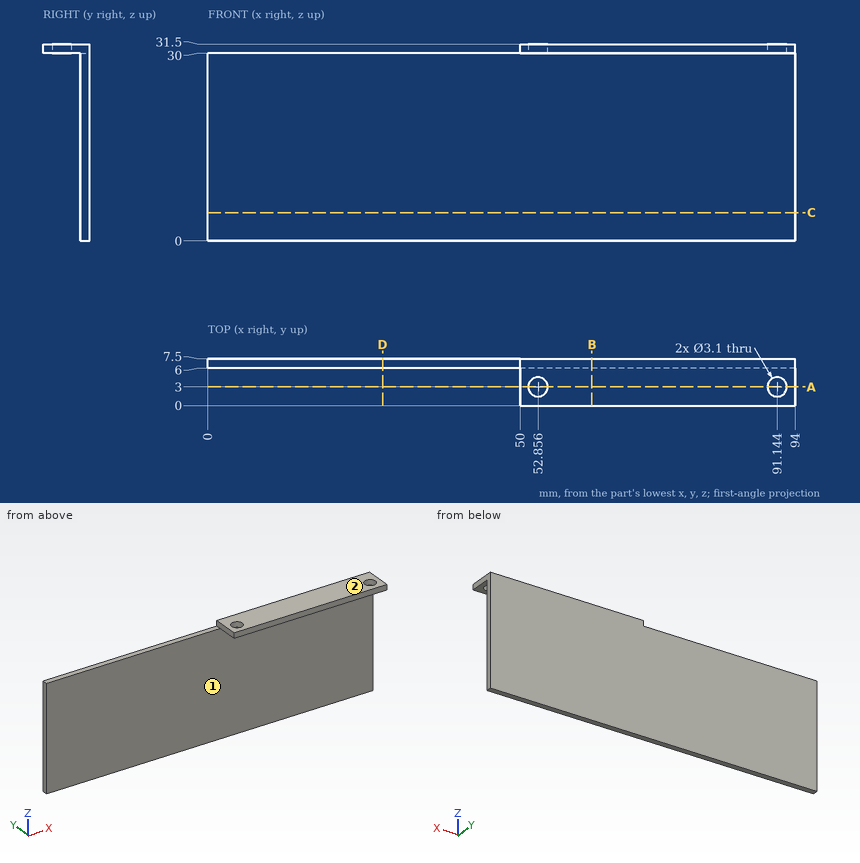
Geometry: see drawing. Coordinates: mm, zero at the bounding-box minimum. A direction names the side the tool comes from. Coordinates: 2 decimals unless noted, no trailing zeros. Loops run counter-clockwise (first coordinate to the right, second up) from the corner with the lowest first, then second, coordinate; pieces in that order, holes last.
(1) Section C-C on z = 4.5. Return the cut outline in (x, y), then the cut area to 3 significant figures.
(2) Set-up query: the marked faces 1 and 2. Return all of +Z, -Z, +X, -X, +Y, -Y with unobstructed straight access to the full face (end or side cutting, diameter ignored); none if empty.
(3) Section B-B on x = 61.5. Return the cut outline in (y, z).
(4) First-contact query: pin 1 Ø2 at (x, y) = (59, 4.5) entering from -Z; pin 2 Ø0.8 at (y, z) = (3, 30.5) entering from -X; pin 3 Ø10 at (x, z) = (26.5, 12.5) entering from -Y. Flat tips, straight axial feed; report the tip coordinate or a pass-through.
(5) Section A-A on y = 3. Return the cut outline in (x, z).
(6) Material intervals for probe 1 along Y at (x, z) = (6, 2.5); probe 2 along Z at (x, y) = (77, 1.5); probe 3 along Z at (x, y) = (22, 6.5), sorted ascending.
(7) Section D-D on x = 28. Return the cut outline in (y, z), then the cut area to 3 significant figures.
Data:
1. outline: (0, 6) - (94, 6) - (94, 7.5) - (0, 7.5) - close
1. area: 141 mm2
2. face 1: -Z, +X, -X, -Y
2. face 2: +Z, +X, -X, +Y, -Y
3. outline: (0, 30) - (6, 30) - (6, 0) - (7.5, 0) - (7.5, 31.5) - (0, 31.5) - close
4. pin 1: stops at z = 30
4. pin 2: stops at x = 50
4. pin 3: stops at y = 6
5. outline: (50, 30) - (51.31, 30) - (51.31, 31.5) - (50, 31.5) - close; (54.41, 30) - (89.59, 30) - (89.59, 31.5) - (54.41, 31.5) - close; (92.69, 30) - (94, 30) - (94, 31.5) - (92.69, 31.5) - close
6. probe 1: y = 6 to 7.5
6. probe 2: z = 30 to 31.5
6. probe 3: z = 0 to 30
7. outline: (6, 0) - (7.5, 0) - (7.5, 30) - (6, 30) - close
7. area: 45.0 mm2
